Work out the finished part from the listing and answer in its coordinate system (mm). Face numbers are marked on the shaded views. A direction names the side the tool comes from. Give positions to 0.01 mm unless a question says otherwise; leave off trailing zeros. Order: outer loops, then holes, each group sorted by start corner. A loop starts at its lowest first (then second) coordinate and runs counter-clockwise, first axis right, second up. Notation, with made-up numbers: (3, 17) - (17, 17) arc R15 cw to (17, 33) - close; hole circle Ø1 at (16, -4.75). An arc over 180 degrees is marked (long way). Put each result on its own line as item: value.
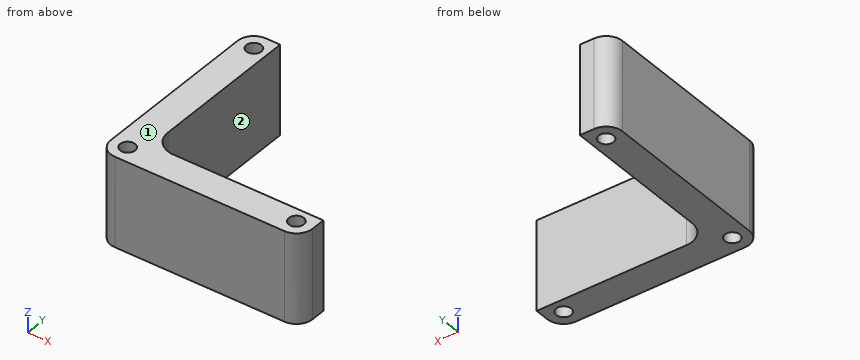
```python
from build123d import *

# Parameters (mm, degrees)
ESQUISSE1_W                               = 56.4
ESQUISSE1_H                               = 56.4
BOSS_EXTRU_1_DEPTH                        = 25
ESQUISSE2_W                               = 75.873546066
ESQUISSE2_H                               = 70.951609501
ENL_V_MAT_EXTRU_1_DEPTH                   = 26
TROU_POUR_TARAUDAGE_POUR_TROU_TARAUD_M5_D = 4.2
CONG_1_R                                  = 6
CONG_2_R                                  = 4.5


with BuildPart() as part:
    # Esquisse1 → Boss.-Extru.1 (new body)
    with BuildSketch(Plane.XY):
        Rectangle(ESQUISSE1_W, ESQUISSE1_H)
    extrude(amount=BOSS_EXTRU_1_DEPTH)

    # Esquisse2 → Enlèv. mat.-Extru.1 (cut, through all)
    with BuildSketch(Plane.XY.offset(25)):
        with Locations((18.236773033, 15.775804751)):
            Rectangle(ESQUISSE2_W, ESQUISSE2_H)
    extrude(amount=-ENL_V_MAT_EXTRU_1_DEPTH, mode=Mode.SUBTRACT)

    # Trou pour taraudage pour trou taraudé M51 (through all)
    with Locations(Plane.XY.offset(25)):
        with Locations((23.57, 23.57), (-23.57, -23.57), (-23.57, 23.57), (23.57, -23.57)):
            Hole(TROU_POUR_TARAUDAGE_POUR_TROU_TARAUD_M5_D / 2)

    # Congé1
    cong_1_edges = [part.edges().sort_by_distance(p)[0] for p in [
        (-19.7, -19.7, 12.5),
    ]]
    fillet(cong_1_edges, radius=CONG_1_R)

    # Congé2
    cong_2_edges = [part.edges().sort_by_distance(p)[0] for p in [
        (28.2, -28.2, 12.5),
        (-28.2, -28.2, 12.5),
        (-28.2, 28.2, 12.5),
    ]]
    fillet(cong_2_edges, radius=CONG_2_R)


solid = part.part
```
(1) Section C-C, the plane x = 14 is taken. Write down the section's boundary in (y, z), then the cut area to 4 significant figures.
Geometry check:
outline: (-28.2, 0) - (-19.7, 0) - (-19.7, 25) - (-28.2, 25) - close
area: 212.5 mm²
(2) Section B-B, the plane y = 24.5 is taken. Write down the section's boundary in (x, z), then the cut area to 3 significant figures.
Geometry check:
outline: (-28.13, 0) - (-25.45, 0) - (-25.45, 25) - (-28.13, 25) - close; (-21.69, 0) - (-19.7, 0) - (-19.7, 25) - (-21.69, 25) - close
area: 117 mm²
(3) A tool of negligible diameter and unlimited length cuts with its end or side. For the marked faces 1 and 2, from which of +Z, -Z, +X, -X, +Y, -Y can it reach the whole face along a straight path? Write none if from no direction.
Geometry check:
face 1: +Z, +X, -X, +Y, -Y
face 2: +Z, -Z, +X, +Y
(4) Section A-A, the plane z = 6.5 is taken. Write down the section's boundary in (x, y).
Geometry check:
outline: (-28.2, -23.7) arc R4.5 ccw to (-23.7, -28.2) - (23.7, -28.2) arc R4.5 ccw to (28.2, -23.7) - (28.2, -19.7) - (-13.7, -19.7) arc R6 cw to (-19.7, -13.7) - (-19.7, 28.2) - (-23.7, 28.2) arc R4.5 ccw to (-28.2, 23.7) - close; hole circle Ø4.2 at (-23.57, -23.57); hole circle Ø4.2 at (-23.57, 23.57); hole circle Ø4.2 at (23.57, -23.57)
(5) Given pin 1 (7.5 mm diameter, centred on y = 7, z = 12, fed in from +X); pin 2 (1.5 mm diameter, centred on x = -13.5, z = 17.5, fed in from +Y), each flat-ended and moving along its own axis, determine where each tip first touches the part or whether it passes through.
Geometry check:
pin 1: stops at x = -19.7
pin 2: stops at y = -19.67
(6) Straight lines are drawn through the part: line 1 (Y direction, x = -23.57, z = 9); line 2 (Y direction, x = -12, z = 10.75); line 3 (Y direction, x = 23.57, z = 16). For each, find the intervals that lie inside material, in ascending order.
Geometry check:
line 1: y = -28.2 to -25.67, -21.47 to 21.47, 25.67 to 28.2
line 2: y = -28.2 to -19.7
line 3: y = -28.2 to -25.67, -21.47 to -19.7
